Study the drawing (mm; zero at the part's minimum x, y, z) and answer. A direction names the side the tool comes from. Coordinates: 2 decimals unless noted, no trailing zeros. Write each loop counter-clockwise with the first axis right and the second up, starting at its lowest first coordinate (ties: lowest second). Pieces come first, ordered by that corner, then holes. Notation, with made-up numbers: M 40,-26 L 81,-26 A32 ccw 81,2 Z; hole C -1,54 d4. An arc over 180 degrees is marked long. Answer as a JSON object with one key per item and string values. Group by question number.
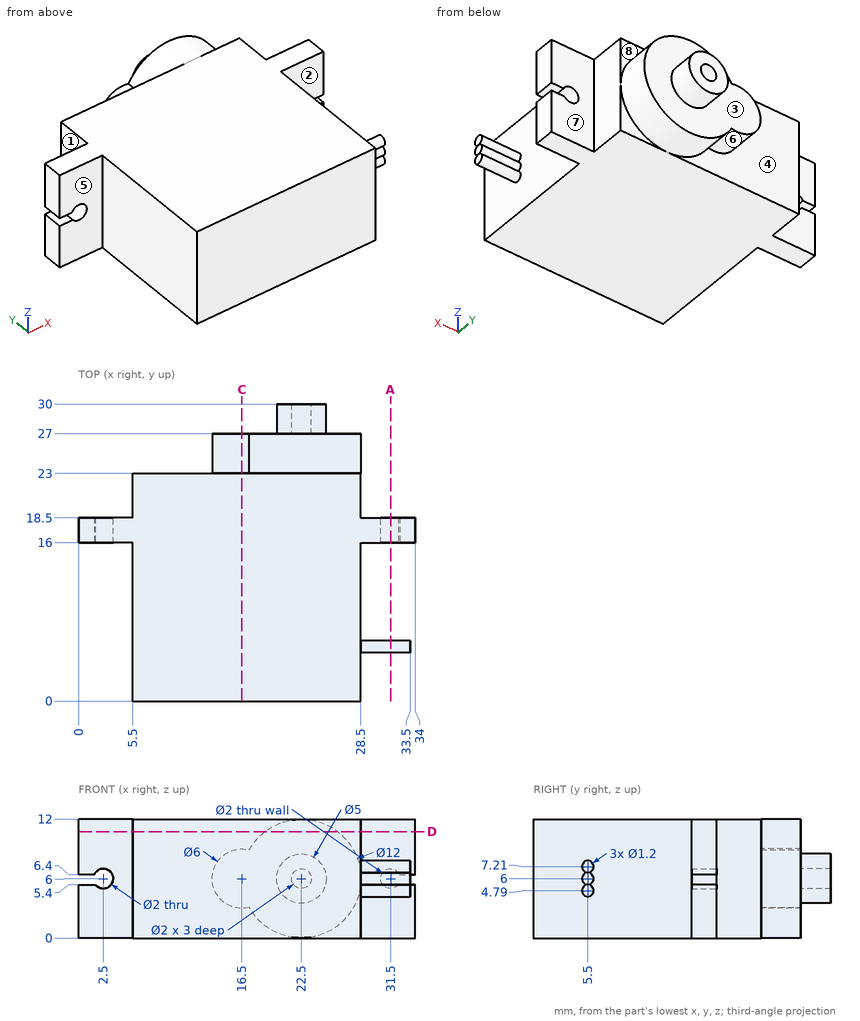
Item 1: A cutting plane is placed at A-A, the plane x = 31.5. Write down the section's boundary in (y, z).
Item 2: A cutting plane is placed at C-C, the plane x = 16.5. Write down the section's boundary in (y, z), and give its area (3 significant figures).
Item 3: A tool of negligible diameter and unlimited length cuts with its end or side. For the marked faces 4, 5, 6, 7 and 8, from which of +Z, -Z, +X, -X, +Y, -Y can it reach the whole face along a straight path? Write none if from no direction.
Item 4: A cutting plane is placed at D-D, the plane z = 10.75. Write down the section's boundary in (x, y), and give its area (3 significant figures).
Item 5: Consider L1, parallel to Y at x = 6, z = 3.75; L2, parallel to Y at x = 24, z = 11.25; L3, parallel to X at y = 17.8, z = 6. Determine where each line is inside the solid, lowest interval first. Write a range as from..to.
Item 6: Flat-ended cylindrical pins translate along their axes: pin 1 Ø1 at (y, z) = (5.5, 6) entering from +X; pin 2 Ø1.8 at (x, z) = (26.5, 4) entering from +Y; pin 3 Ø1 at (y, z) = (12, 8) entering from +X. Find the tip coordinate at first contact, or state that the pin passes through.
Item 7: For a pull along Y with two mould halves and no side action, classify the marked faces 1, 2 and 3 as +Y half, -Y half, draft (parallel to the pull), parting line (faces both ways), or undercut.
Answer:
{
 "1": {"outline": "C 5.5,4.79 d1.2; C 5.5,6 d1.2; C 5.5,7.21 d1.2; M 16,0 L 18.5,0 L 18.5,5 L 16,5 Z; M 16,7 L 18.5,7 L 18.5,12 L 16,12 Z"},
 "2": {"outline": "M 0,0 L 23,0 L 23,3 L 27,3 L 27,9 L 23,9 L 23,12 L 0,12 Z", "area": "300 mm2"},
 "3": {"face 4": "-X, +Y", "face 5": "+Z, -Z, -X, -Y", "face 6": "+Y", "face 7": "+Z, -Z, +X, +Y", "face 8": "+Z, +X, +Y"},
 "4": {"outline": "M 0,16 L 5.5,16 L 5.5,0 L 28.5,0 L 28.5,16 L 34,16 L 34,18.5 L 28.5,18.5 L 28.5,23 L 26.17,23 L 26.17,27 L 18.83,27 L 18.83,23 L 5.5,23 L 5.5,18.5 L 0,18.5 Z", "area": "586 mm2"},
 "5": {"L1": "0..23", "L2": "0..27", "L3": "3.5..30.5"},
 "6": {"pin 1": "x = 33.5", "pin 2": "y = 27", "pin 3": "x = 28.5"},
 "7": {"face 1": "draft", "face 2": "undercut", "face 3": "+Y half"}
}
